Part model, mm, in its own coordinate system. Face numbers are marked on the shaded views. A direction names the side the tool comes from. Coordinates: 2 decimals unless noted, no trailing zeros. Loops run counter-clockwise (first coordinate to the right, second up) from the corner with the lowest first, then second, coordinate; pieces in that order, holes last. Notation, with made-up numbers: (53.5, 75) - (99.5, 75) arc R27 ccw to (99.5, 103) - close; hole circle Ø9 at (68, 72.25). An arc over 180 degrees is marked (long way). Answer as CSV lines item,"result".
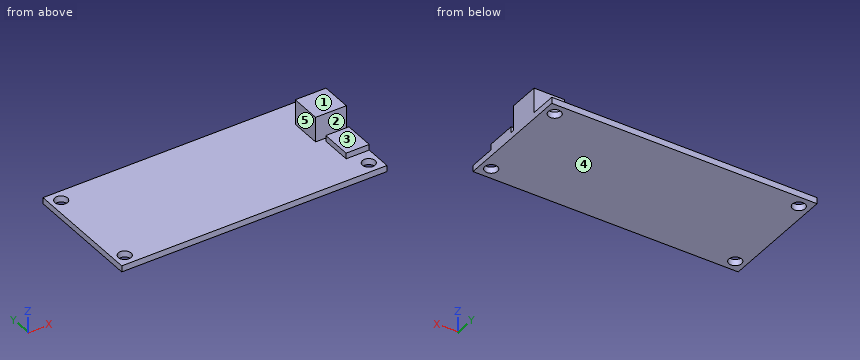
Autodesk Inventor part; units mm, degrees
ref_plane "YZ Plane" through (0, 0, 0) normal (1, 0, 0) x (0, 1, 0)
ref_plane "XZ Plane" through (0, 0, 0) normal (0, 1, 0) x (-1, 0, 0)
ref_plane "XY Plane" through (0, 0, 0) normal (0, 0, 1) x (1, 0, 0)
sketch "Skizze1" plane through (0, 0, 0) normal (0, 0, 1) x (1, 0, 0)
  line L0 (-13.8, 0) -> (82.8, 0)
  line L1 (0, -6.2) -> (0, 37.2)
  line L2 (0, 0) -> (69, 0)
  line L3 (69, 0) -> (69, 31)
  line L4 (69, 31) -> (0, 31)
  line L5 (0, 31) -> (0, 0)
  line L6 (2.75, 28) -> (66.25, 28) construction
  line L7 (66.25, 28) -> (66.25, 3) construction
  line L8 (66.25, 3) -> (2.75, 3) construction
  line L9 (2.75, 3) -> (2.75, 28) construction
  circle A0 centre (2.75, 28) radius 1.65
  circle A1 centre (2.75, 3) radius 1.65
  circle A2 centre (66.25, 28) radius 1.65
  circle A3 centre (66.25, 3) radius 1.65
  dimension "d0" = 31
  dimension "d1" = 69
  dimension "d4" = 25
  dimension "d5" = 63.5
  dimension "d6" = 2.75
  dimension "d7" = 3
  dimension "d8" = 3.3
extrude "Extrusion2" add sketch "Skizze1" along normal blind 1.6
sketch "Skizze2" plane through (0, 0, 1.6) normal (0, 0, 1) x (1, 0, 0)
  line L0 (69, 0) -> (69, 31)
  line L1 (69, 31) -> (0, 31)
  line L2 (69, 16) -> (61, 16)
  line L3 (61, 16) -> (61, 24)
  line L4 (61, 24) -> (69, 24)
  line L5 (69, 24) -> (69, 16)
  dimension "d11" = 15
  dimension "d12" = 8
  dimension "d13" = 8
extrude "Extrusion3" add sketch "Skizze2" along normal blind 6.5
sketch "Skizze3" plane through (0, 0, 1.6) normal (0, 0, 1) x (1, 0, 0)
  line L0 (0, 0) -> (69, 0)
  line L1 (69, 0) -> (69, 16)
  line L2 (69, 15) -> (63, 15)
  line L3 (63, 15) -> (63, 7)
  line L4 (63, 7) -> (69, 7)
  line L5 (69, 7) -> (69, 15)
  dimension "d16" = 8
  dimension "d17" = 6
  dimension "d18" = 15
extrude "Extrusion4" add sketch "Skizze3" along normal blind 1.5
properties part number "IOIO Board"
Q1. Saw through at B-B (x = 66.25). Give the cut face in (y, z).
Results:
outline,"(0, 0) - (1.35, 0) - (1.35, 1.6) - (0, 1.6) - close; (4.65, 0) - (26.35, 0) - (26.35, 1.6) - (24, 1.6) - (24, 8.1) - (16, 8.1) - (16, 1.6) - (15, 1.6) - (15, 3.1) - (7, 3.1) - (7, 1.6) - (4.65, 1.6) - close; (29.65, 0) - (31, 0) - (31, 1.6) - (29.65, 1.6) - close"
Q2. Saw through at C-C (y = 20.5). Give the cut face in (x, z), then the cut area to 3 significant figures.
Results:
outline,"(0, 0) - (69, 0) - (69, 8.1) - (61, 8.1) - (61, 1.6) - (0, 1.6) - close"
area,"162 mm^2"
Q3. Two-plate mould, pull along Y, no slides. Class the marked faces 1 and 2: released by +Y, released by -Y, zero draft, split by the parting line, or undercut.
Results:
face 1,"zero draft"
face 2,"undercut"
Q4. Flat gauge pins, fed straight in: pin 1 (0.8 mm diameter, centred on x = 67.5, z = 2.5, fed in from +Y); pin 2 (3 mm diameter, centred on x = 23.5, y = 17.5, fed in from +Z); pin 3 (0.8 mm diameter, centred on x = 67, z = 2.5, fed in from -Y). Where does each tip first touch, or does it go through?
Results:
pin 1,"stops at y = 24"
pin 2,"stops at z = 1.6"
pin 3,"stops at y = 7"
Q5. Which spindle directions (+Z, -Z, +X, -X, +Y, -Y) get a long thin tool onto all of the face, cutting with end or side? Do the marked faces 3, 4 and 5. Say none if no direction does.
Results:
face 3,"+Z, +X, -X, -Y"
face 4,"-Z, +X, -X, +Y, -Y"
face 5,"+Z, -X, +Y, -Y"
Q6. Wall check: L1, parallel to Y at x = 66.25, z = 0.7; L2, parallel to Z at x = 29.5, y = 9.5; L3, parallel to X at y = 17, z = 3. Give the ranges that are in metal, low to high.
Results:
L1,"y = 0 to 1.35, 4.65 to 26.35, 29.65 to 31"
L2,"z = 0 to 1.6"
L3,"x = 61 to 69"
Q7. Saw through at D-D (x = 2.75). Give the cut face in (y, z).
Results:
outline,"(0, 0) - (1.35, 0) - (1.35, 1.6) - (0, 1.6) - close; (4.65, 0) - (26.35, 0) - (26.35, 1.6) - (4.65, 1.6) - close; (29.65, 0) - (31, 0) - (31, 1.6) - (29.65, 1.6) - close"
Q8. Saw through at A-A (y = 28). Give the cut face in (x, z).
Results:
outline,"(0, 0) - (1.1, 0) - (1.1, 1.6) - (0, 1.6) - close; (4.4, 0) - (64.6, 0) - (64.6, 1.6) - (4.4, 1.6) - close; (67.9, 0) - (69, 0) - (69, 1.6) - (67.9, 1.6) - close"
